Design review of the part built by this model. Coordinates are the model's own, in mm. Face numbers are marked on the shaded views. A direction names the side the tool comes from. Round coordinates to 2 decimals unless told otherwise and drop trailing zeros. Write each loop counter-clockwise with the first axis right and the second up, starting at its lowest first coordinate (ties: lowest second). Pieces come first, ordered by that corner, then holes. Notation, with made-up numbers: M 53,38.25 L 100,38.25 A16 ccw 100,65.25 Z; hole C 42.5,-37 d5. An arc over 180 degrees is marked long. Use CSV: the item, a comma, the result in double quotes.
from build123d import *

# Parameters (mm, degrees)
CROQUIS1_R              = 25.4
SALIENTE_EXTRUIR1_DEPTH = 7.9375
CROQUIS2_W              = 70
CROQUIS2_H              = 115
CROQUIS2_R              = 6.35
SALIENTE_EXTRUIR2_DEPTH = 7.9375


with BuildPart() as part:
    # Croquis1 → Saliente-Extruir1 (new body)
    with BuildSketch(Plane.XY):
        with BuildLine():
            Line((-35, 72.154), (-35, 0))
            Line((-35, 0), (35, 0))
            Line((35, 0), (35, 72.154))
            ThreePointArc((35, 72.154), (24.903139014, 97.889287059), (0, 109.89283941))
            ThreePointArc((0, 109.89283941), (-24.903139014, 97.889287059), (-35, 72.154))
        make_face()
        with Locations((0, 72.9)):
            Circle(CROQUIS1_R, mode=Mode.SUBTRACT)
    extrude(amount=SALIENTE_EXTRUIR1_DEPTH)

    # Croquis2 → Saliente-Extruir2 (add)
    with BuildSketch(Plane.XZ):
        with Locations((0, 57.5)):
            Rectangle(CROQUIS2_W, CROQUIS2_H)
        with Locations(Location((-0.254, 35.772581169, 0), (0, 0, 270))):
            Circle(CROQUIS2_R, mode=Mode.SUBTRACT)
        with Locations(Location((0, 95.772581169, 0), (0, 0, 270))):
            Circle(CROQUIS2_R, mode=Mode.SUBTRACT)
    extrude(amount=-SALIENTE_EXTRUIR2_DEPTH)


solid = part.part
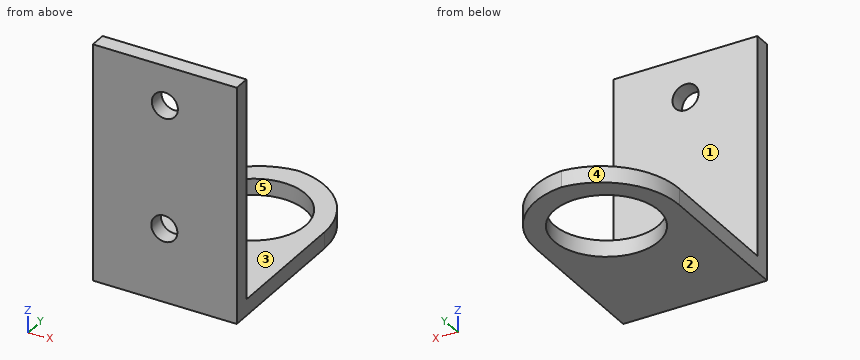
1) The part is to be moulded in two halves that separate along Y. For the marked faces 3, 4 and 5, say which applies: released by +Y, released by -Y, zero draft, split by the parting line, or undercut.
Answers:
face 3,"zero draft"
face 4,"released by +Y"
face 5,"undercut"
2) Add section C-C on z = 32.5. Write out the cut boundary in (x, y), then the cut area to 3 significant figures.
Answers:
outline,"M -35,0 L -5.7,0 L -5.7,7.94 L -35,7.94 Z; M 5.19,0 L 35,0 L 35,7.94 L 5.19,7.94 Z"
area,"469 mm²"
3) Wall thickness on line 1 along Y through (x, z) = (0, 3); line 2 along Y through (x, z) = (18, 26.5): over which ranges is each line inside the solid? List them lowest first. Write a range as [from, to].
Answers:
line 1,"[0, 47.5], [98.3, 109.89]"
line 2,"[0, 7.94]"
4) Machinability: for the marked faces 1 and 2, which of the approach directions +Z, -Z, +X, -X, +Y, -Y give a long, thin tool a straight path to every point of the face, cutting with its end or side? Answer none if there is none.
Answers:
face 1,"+Z, +X, -X, +Y"
face 2,"-Z, +X, -X, +Y, -Y"
5) Add section D-D on x = 4. Write out the cut boundary in (y, z).
Answers:
outline,"M 0,0 L 47.82,0 L 47.82,7.94 L 7.94,7.94 L 7.94,31.06 L 0,31.06 Z; M 0,40.49 L 7.94,40.49 L 7.94,90.84 L 0,90.84 Z; M 0,100.7 L 7.94,100.7 L 7.94,115 L 0,115 Z; M 97.98,0 L 109.38,0 L 109.38,7.94 L 97.98,7.94 Z"
6) For pin 1 Ø20.5 at (x, z) = (-0.25, 35.77) entering from +Y, flat-tipped, find the tip position at first contact; note if it passes through.
Answers:
pin 1,"y = 7.94"
7) Add section A-A on y = 54.5. Write out the cut boundary in (x, z), then the cut area to 3 significant figures.
Answers:
outline,"M -35,0 L -17.51,0 L -17.51,7.94 L -35,7.94 Z; M 17.51,0 L 35,0 L 35,7.94 L 17.51,7.94 Z"
area,"278 mm²"
8) Add section B-B on x = 19.5. Write out the cut boundary in (y, z), then the cut area to 3 significant figures.
Answers:
outline,"M 0,0 L 56.62,0 L 56.62,7.94 L 7.94,7.94 L 7.94,115 L 0,115 Z; M 89.18,0 L 102.7,0 L 102.7,7.94 L 89.18,7.94 Z"
area,"1,410 mm²"
